Geometry check sheet. Reference: the model listing, model coordinates, mm. A direction names the side the tool comes from. Coordinates: 2 decimals unless noted, no trailing zeros. Write each loop counter-clockwise with the first axis right and the second up, starting at its lowest first coordinate (ties: lowest second). Pieces come first, ordered by that corner, then holes. Notation, with made-up numbers: M 76,27.25 L 93,27.25 A25 cw 93,61.25 Z; hole C 49.25,-5 d5. An arc over 180 degrees is marked long. Write item = value, one per line. Start each with the question number.
```python
from build123d import *

# Parameters (mm, degrees)
SKETCH1_R           = 12.7
BOSS_EXTRUDE1_DEPTH = 2.54
BOSS_EXTRUDE2_DEPTH = 25.4
BOSS_EXTRUDE3_REACH = 19.018
SKETCH3_W           = 6.393920166
SKETCH3_H           = 6.393920167
SKETCH4_R           = 1.397
CUT_EXTRUDE1_DEPTH  = 5.588
CUT_EXTRUDE2_REACH  = 29.94
SKETCH6_R           = 1
CUT_EXTRUDE4_DEPTH  = 1.27
SKETCH10_W          = 3.153039917
SKETCH10_H          = 3.048
BOSS_EXTRUDE4_DEPTH = 10.16
CHAMFER1_SIZE       = 1.27
BOSS_EXTRUDE5_DEPTH = 2.54


with BuildPart() as part:
    # Sketch1 → Boss-Extrude1 (new body)
    with BuildSketch(Plane(origin=(0, 0, 0), x_dir=(1, 0, 0), z_dir=(0, 1, 0))):
        Circle(SKETCH1_R)
    extrude(amount=BOSS_EXTRUDE1_DEPTH)

    # Sketch2 → Boss-Extrude2 (add)
    with BuildSketch(Plane(origin=(0, 2.54, 0), x_dir=(1, 0, 0), z_dir=(0, 1, 0))):
        with BuildLine():
            Line((12.516478449, -2.151224589), (-12.516478449, -2.151224589))
            ThreePointArc((-12.516478449, -2.151224589), (-12.187390109, -3.571767395), (-11.697638811, -4.945224589))
            Line((-11.697638811, -4.945224589), (11.697638811, -4.945224589))
            ThreePointArc((11.697638811, -4.945224589), (12.187390109, -3.571767395), (12.516478449, -2.151224589))
        make_face()
    extrude(amount=BOSS_EXTRUDE2_DEPTH)

    # Sketch3 → Boss-Extrude3 (add, up to next)
    with BuildSketch(Plane(origin=(0, 0, -4.318), x_dir=(-1, 0, 0), z_dir=(0, 0, -1)), mode=Mode.PRIVATE) as boss_extrude3_sk1:
        with Locations((0, 24.743039917)):
            Rectangle(SKETCH3_W, SKETCH3_H)
    boss_extrude3_tool1 = extrude(boss_extrude3_sk1.sketch, amount=-BOSS_EXTRUDE3_REACH, mode=Mode.PRIVATE) - part.part
    add(boss_extrude3_tool1.solids().sort_by_distance((0, 24.74304, -4.318))[0])

    # Sketch4 → Cut-Extrude1 (cut)
    with BuildSketch(Plane(origin=(0, 0, -4.318), x_dir=(-1, 0, 0), z_dir=(0, 0, -1))):
        with Locations((0, 24.743039917)):
            Circle(SKETCH4_R)
    extrude(amount=-CUT_EXTRUDE1_DEPTH, mode=Mode.SUBTRACT)

    # Sketch6 → Cut-Extrude2 (cut, up to next)
    with BuildSketch(Plane.XZ, mode=Mode.PRIVATE) as cut_extrude2_sk1:
        with Locations((9, 0)):
            Circle(SKETCH6_R)
    cut_extrude2_tool1 = extrude(cut_extrude2_sk1.sketch, amount=-CUT_EXTRUDE2_REACH, mode=Mode.PRIVATE) & part.part
    add(cut_extrude2_tool1.solids().sort_by_distance((9, 0, 0))[0], mode=Mode.SUBTRACT)
    # Sketch6 → Cut-Extrude2 (cut, up to next)
    with BuildSketch(Plane.XZ, mode=Mode.PRIVATE) as cut_extrude2_sk2:
        with Locations((0, -6.6)):
            Circle(SKETCH6_R)
    cut_extrude2_tool2 = extrude(cut_extrude2_sk2.sketch, amount=-CUT_EXTRUDE2_REACH, mode=Mode.PRIVATE) & part.part
    add(cut_extrude2_tool2.solids().sort_by_distance((0, 0, -6.6))[0], mode=Mode.SUBTRACT)
    # Sketch6 → Cut-Extrude2 (cut, up to next)
    with BuildSketch(Plane.XZ, mode=Mode.PRIVATE) as cut_extrude2_sk3:
        with Locations((-9, 0)):
            Circle(SKETCH6_R)
    cut_extrude2_tool3 = extrude(cut_extrude2_sk3.sketch, amount=-CUT_EXTRUDE2_REACH, mode=Mode.PRIVATE) & part.part
    add(cut_extrude2_tool3.solids().sort_by_distance((-9, 0, 0))[0], mode=Mode.SUBTRACT)
    # Sketch6 → Cut-Extrude2 (cut, up to next)
    with BuildSketch(Plane.XZ, mode=Mode.PRIVATE) as cut_extrude2_sk4:
        with Locations((0, 6.6)):
            Circle(SKETCH6_R)
    cut_extrude2_tool4 = extrude(cut_extrude2_sk4.sketch, amount=-CUT_EXTRUDE2_REACH, mode=Mode.PRIVATE) & part.part
    add(cut_extrude2_tool4.solids().sort_by_distance((0, 0, 6.6))[0], mode=Mode.SUBTRACT)
    # Sketch6 → Cut-Extrude2 (cut, up to next)
    with BuildSketch(Plane.XZ, mode=Mode.PRIVATE) as cut_extrude2_sk5:
        Circle(SKETCH6_R)
    cut_extrude2_tool5 = extrude(cut_extrude2_sk5.sketch, amount=-CUT_EXTRUDE2_REACH, mode=Mode.PRIVATE) & part.part
    add(cut_extrude2_tool5.solids().sort_by_distance((0, 0, 0))[0], mode=Mode.SUBTRACT)

    # Sketch9 → Cut-Extrude4 (cut)
    with BuildSketch(Plane.XZ):
        with BuildLine():
            Line((-2.1, -6.6), (-2.1, -3.046309242))
            ThreePointArc((-2.1, -3.046309242), (-2.376743942, -2.835681264), (-2.632489316, -2.6))
            Line((-2.632489316, -2.6), (-3.60208243, -2.6))
            Line((-3.60208243, -2.6), (-15.602107818, -2.099998942))
            ThreePointArc((-15.602107818, -2.099998942), (-17.7, 0), (-15.602107818, 2.099998942))
            Line((-15.602107818, 2.099998942), (-3.60208243, 2.6))
            Line((-3.60208243, 2.6), (-2.632489316, 2.6))
            ThreePointArc((-2.632489316, 2.6), (-2.376743942, 2.835681264), (-2.1, 3.046309242))
            Line((-2.1, 3.046309242), (-2.1, 6.6))
            ThreePointArc((-2.1, 6.6), (0, 8.7), (2.1, 6.6))
            Line((2.1, 6.6), (2.1, 3.046309242))
            ThreePointArc((2.1, 3.046309242), (2.376743942, 2.835681264), (2.632489316, 2.6))
            Line((2.632489316, 2.6), (3.60208243, 2.6))
            Line((3.60208243, 2.6), (15.602107818, 2.099998942))
            ThreePointArc((15.602107818, 2.099998942), (17.7, 0), (15.602107818, -2.099998942))
            Line((15.602107818, -2.099998942), (3.60208243, -2.6))
            Line((3.60208243, -2.6), (2.632489316, -2.6))
            ThreePointArc((2.632489316, -2.6), (2.376743942, -2.835681264), (2.1, -3.046309242))
            Line((2.1, -3.046309242), (2.1, -6.6))
            ThreePointArc((2.1, -6.6), (0, -8.7), (-2.1, -6.6))
        make_face()
    extrude(amount=-CUT_EXTRUDE4_DEPTH, mode=Mode.SUBTRACT)

    # Sketch10 → Boss-Extrude4 (add)
    with BuildSketch(Plane(origin=(0, 0, 2.151224589), x_dir=(-1, 0, 0), z_dir=(0, 0, -1))):
        with Locations((-4.773480042, 24.416)):
            Rectangle(SKETCH10_W, SKETCH10_H)
        with Locations((4.773480042, 24.416)):
            Rectangle(SKETCH10_W, SKETCH10_H)
    extrude(amount=BOSS_EXTRUDE4_DEPTH)

    # Chamfer1
    chamfer1_edges = [part.edges().sort_by_distance(p)[0] for p in [
        (4.773480042, 22.892, 2.151224589),
        (-4.773480042, 22.892, 2.151224589),
        (0, 21.546079833, 2.151224589),
    ]]
    chamfer(chamfer1_edges, length=CHAMFER1_SIZE)

    # Sketch11 → Boss-Extrude5 (add)
    with BuildSketch(Plane(origin=(0, 2.54, 0), x_dir=(1, 0, 0), z_dir=(0, 1, 0))):
        with BuildLine():
            Line((-6.35, 10.998522628), (6.35, 10.998522628))
            ThreePointArc((6.35, 10.998522628), (0, 12.7), (-6.35, 10.998522628))
        make_face()
    extrude(amount=BOSS_EXTRUDE5_DEPTH)


solid = part.part
```
Q1. Cross-section at D-D on x = 9. Enter the section's corners in (y, z), and give its area (3 significant figures).
Q2. Gauge pin test, flat ends, axial feed: pin 1 (4 mm diameter, centred on y = 21, z = -3.5, fed in from -X); pin 2 (0.9 mm diameter, centred on x = -1, z = -12, fed in from +Y); pin 3 (3 mm diameter, centred on x = 8.5, z = -8.5, fed in from -Y); pin 4 (4 mm diameter, centred on y = 19, z = 6.5, fed in from -X). Record the tip position at first contact, or that the pin passes through.
Q3. Set-up check for faces 4 (the face through (3.197, 27, -1)), 5 (the face through (2.1, 1, -5)), 6 (the face through (4.796, 22.248, 1.525)): record each of +Z, -Z, +X, -X, +Y, -Y from which the full face is reachable in a straight line by a thin tool's end or side.
Q4. Scan lines: L1, parallel to Y at x = 0, z = -1.7; L2, parallel to Z at x = 0, y = 1.85; L3, parallel to Y at x = -3.75, z = -6.5. Record each from-to range of solid material in increasing order.
Q5. Cross-section at B-B on x = 0. Count the separate pieces of the cut face and the enclosed holes in it, and give its area (3 significant figures).
Q6. Cross-section at C-C on y = 24.25. Enter the section's corners in (x, z).
Q7. Draft check along Z on faces 1 (the face through (5, 24, -8.009)), 2 (the face through (-5, 22.892, -4)), 3 (the face through (-9.8, 1.9, -0.6)). Enter one of: pulls with the +Z half, pulls with the -Z half, needs draft (parallel to the pull), parting line crosses it, or undercut.
Q8. Cross-section at A-A on z = -3.5. Enter the section's corners in (x, y).
Values found:
q1.outline = M 0,-8.96 L 2.54,-8.96 L 2.54,-1 L 1.27,-1 L 1.27,-2.38 L 0,-2.38 Z; M 0,2.38 L 1.27,2.38 L 1.27,1 L 2.54,1 L 2.54,2.15 L 27.94,2.15 L 27.94,4.95 L 2.54,4.95 L 2.54,8.96 L 0,8.96 Z
q1.area = 108 mm²
q2.pin_1 = -6.35
q2.pin_2 = 5.08
q2.pin_3 = 0
q2.pin_4 = -11.88
q3.face_4 = -Z, +X, +Y
q3.face_5 = -Y
q3.face_6 = -Z, +X
q4.L1 = 1.27 to 2.54, 21.55 to 23.35, 26.14 to 27.94
q4.L2 = -12.7 to -7.6, -5.6 to -1, 1 to 5.6, 7.6 to 12.7
q4.L3 = 0 to 2.54, 22.89 to 25.94
q5.separate_pieces = 4
q5.enclosed_holes = 0
q5.area = 137 mm²
q6.outline = M -12.52,2.15 L -6.35,2.15 L -6.35,-8.01 L -3.2,-8.01 L -3.2,-4.32 L -1.31,-4.32 L -1.31,1.27 L 1.31,1.27 L 1.31,-4.32 L 3.2,-4.32 L 3.2,-8.01 L 6.35,-8.01 L 6.35,2.15 L 12.52,2.15 A12.7 ccw 11.7,4.95 L -11.7,4.95 A12.7 ccw Z
q7.face_1 = pulls with the -Z half
q7.face_2 = needs draft
q7.face_3 = undercut
q8.outline = M -12.21,0 L -2.1,0 L -2.1,1.27 L 2.1,1.27 L 2.1,0 L 12.21,0 L 12.21,2.54 L -12.21,2.54 Z; M -6.35,22.89 L -3.2,22.89 L -3.2,21.55 L 3.2,21.55 L 3.2,22.89 L 6.35,22.89 L 6.35,25.94 L 3.2,25.94 L 3.2,27.94 L -3.2,27.94 L -3.2,25.94 L -6.35,25.94 Z; hole C 0,24.74 d2.79
